Source: CAD feature listing. Evaluate the final solid. Frame: model axes, mm. A direction names the side the tool comes from. Round coordinates to 2 decimals unless told otherwise and drop trailing zeros. Order: outer loops, then holes, each group sorted by start corner. A loop starts at its lowest first (then second) coordinate and runs counter-clockwise, first axis right, second up. Notation, with made-up numbers: (82.25, 21) - (113.25, 21) arc R26 cw to (113.25, 35) - close; hole circle Ø9 at (46, 42). An arc over 180 degrees is marked (long way). Put each result on its own line as item: value. Start each with the question number.
1) Section C-C on x = -8.5. Output: boundary loops of the cut face in (y, z).
2) Section B-B on y = 16. Output: boundary loops of the cut face in (x, z), then the cut area to 3 significant figures.
3) Section A-A on z = -3.5. Output: boundary loops of the cut face in (x, y), then the cut area to 3 significant figures.
4) Line query: probe 1 along Y at (x, z) = (-21, -25); probe 2 along X at (y, z) = (8, -30); probe 3 along Z at (x, y) = (3.5, 23). Output: solid intervals per line, ascending. Write a range as [from, to].
5) Section D-D on y = 8.5. Output: boundary loops of the cut face in (x, z), then the cut area to 3 significant figures.
6) Contact query for flat-ended pins moving along their axis: P1, Ø4, axis at x = -30.5, y = 7, coming from the +Z side; P2, Ø0.9, axis at y = 30.5, z = -34, coming from the -X side; P3, Ø1, axis at x = -9, z = -30, coming from the +Y side. Output: stop coordinate, or through.
7) Access query for faces 1 (the face through (2.46, 26.74, -9.06)), 2 (the face through (-3, 30, -25)), 3 (the face through (-35, 14, -25)). Directions: +Z, -Z, +X, -X, +Y, -Y. A direction counts if a zero-diameter tool reaches every point of the face in a straight line with its end or side. Return the directions, or none.
Autodesk Inventor part; units mm, degrees
ref_plane "YZ Plane" through (0, 0, 0) normal (1, 0, 0) x (0, 1, 0)
ref_plane "XZ Plane" through (0, 0, 0) normal (0, 1, 0) x (-1, 0, 0)
ref_plane "XY Plane" through (0, 0, 0) normal (0, 0, 1) x (1, 0, 0)
sketch "Sketch1" plane through (0, 0, 0) normal (0, 1, 0) x (-1, 0, 0)
  line L0 (0, 0) -> (35, 0)
  line L1 (35, 0) -> (35, -50)
  line L2 (35, -50) -> (0, -50)
  line L3 (0, -50) -> (0, 0)
  dimension "d0" = 35
  dimension "d1" = 50
extrude "Extrusion1" add sketch "Sketch1" along normal blind 29
sketch "Sketch2" plane through (0, 29, 0) normal (0, 1, 0) x (1, 0, 0)
  line L0 (0, 50) -> (-35, 50)
  line L1 (0, 0) -> (-3, 0)
  line L2 (-3, 0) -> (-3, 50)
  line L3 (-3, 50) -> (0, 50)
  line L4 (0, 50) -> (0, 0)
  dimension "d4" = 3
extrude "Extrusion2" add sketch "Sketch2" along normal blind 3
sketch "Sketch3" plane through (0, 0, 0) normal (1, 0, 0) x (0, 0, -1)
  circle A0 centre (11.443, 16) radius 11
  dimension "d7" = 22
extrude "Extrusion3" add sketch "Sketch3" along normal blind 5
properties part number "motor"
Answer sheet:
1. outline: (0, -50) - (29, -50) - (29, 0) - (0, 0) - close
2. outline: (-35, -50) - (0, -50) - (0, -22.44) - (5, -22.44) - (5, -0.44) - (0, -0.44) - (0, 0) - (-35, 0) - close
2. area: 1,860 mm^2
3. outline: (-35, 0) - (0, 0) - (0, 8.39) - (5, 8.39) - (5, 23.61) - (0, 23.61) - (0, 32) - (-3, 32) - (-3, 29) - (-35, 29) - close
3. area: 1,100 mm^2
4. probe 1: [0, 29]
4. probe 2: [-35, 0]
4. probe 3: [-19.93, -2.96]
5. outline: (-35, -50) - (0, -50) - (0, -19.49) - (5, -19.49) - (5, -3.4) - (0, -3.4) - (0, 0) - (-35, 0) - close
5. area: 1,830 mm^2
6. P1: z = 0
6. P2: x = -3
6. P3: y = 29
7. face 1: +X
7. face 2: +Z, -Z, -X, +Y
7. face 3: +Z, -Z, -X, +Y, -Y
